```python
from build123d import *

# Parameters (mm, degrees)
AUFSATZ_LINEAR_AUSTRAGEN1_DEPTH             = 350
AUFSATZ_LINEAR_AUSTRAGEN1_DEPTH_BACK        = 350
SKIZZE1_W                                   = 200
SKIZZE1_H                                   = 2166
VERRUNDUNG1_R                               = 400
SKIZZE2_W                                   = 450
SKIZZE2_H                                   = 1500
SCHNITT_LINEAR_AUSTRAGEN1_DEPTH             = 200
SKIZZE4_W                                   = 80
SKIZZE4_H                                   = 1500
SCHNITT_LINEAR_AUSTRAGEN2_DEPTH             = 40
SKIZZE5_R                                   = 40
AUFSATZ_LINEAR_AUSTRAGEN2_DEPTH             = 1500
VERRUNDUNG2_R                               = 10
SKIZZE6_W                                   = 30
SKIZZE6_H                                   = 500
AUFSATZ_LINEAR_AUSTRAGEN3_DEPTH             = 500
SKIZZE7_W                                   = 1200
SKIZZE7_H                                   = 700
AUFSATZ_LINEAR_AUSTRAGEN4_DEPTH             = 10
SCHNITT_LINEAR_AUSTRAGEN3_DEPTH             = 2352.164614527
SCHNITT_LINEAR_AUSTRAGEN4_REACH             = 2264.149
SKIZZE10_W                                  = 160
SKIZZE10_H                                  = 700
SCHNITT_LINEAR_AUSTRAGEN4_DIRECTION_2_DEPTH = 2263.148932027


with BuildPart() as part:
    # Skizze1 → Aufsatz-Linear austragen1 (new, two sides: drawn at the far end of the back side and taken through both)
    with BuildSketch(Plane.XY.offset(-AUFSATZ_LINEAR_AUSTRAGEN1_DEPTH_BACK)):
        with Locations((0, 1083)):
            Rectangle(SKIZZE1_W, SKIZZE1_H)
    extrude(amount=AUFSATZ_LINEAR_AUSTRAGEN1_DEPTH + AUFSATZ_LINEAR_AUSTRAGEN1_DEPTH_BACK)

    # Verrundung1
    # the kernel refuses this fillet: 400 mm, written as the material it takes off along each edge
    with BuildSketch(Plane(origin=(1100, 2166, -350), x_dir=(0, -1, 0), z_dir=(-1, 0, 0)), Plane(origin=(1100, 2166, 350), x_dir=(0, 0, -1), z_dir=(-1, 0, 0))) as verrundung1_piece_1:
        with BuildLine():
            CenterArc((VERRUNDUNG1_R, VERRUNDUNG1_R), VERRUNDUNG1_R, 180, 90)
            Line((0, VERRUNDUNG1_R), (0, 0))
            Line((0, 0), (VERRUNDUNG1_R, 0))
        make_face()
    extrude(amount=2200, mode=Mode.SUBTRACT)

    # Skizze2 → Schnitt-Linear austragen1 (cut)
    with BuildSketch(Plane(origin=(100, 0, 0), x_dir=(0, 0, -1), z_dir=(1, 0, 0))):
        with Locations((0, 1050)):
            Rectangle(SKIZZE2_W, SKIZZE2_H)
    extrude(amount=-SCHNITT_LINEAR_AUSTRAGEN1_DEPTH, mode=Mode.SUBTRACT)

    # Skizze4 → Schnitt-Linear austragen2 (cut)
    with BuildSketch(Plane.XY.offset(-225)):
        with Locations((0, 1050)):
            Rectangle(SKIZZE4_W, SKIZZE4_H)
    schnitt_linear_austragen2 = extrude(amount=-SCHNITT_LINEAR_AUSTRAGEN2_DEPTH, mode=Mode.SUBTRACT)

    # Spiegeln1: Schnitt-Linear austragen2 across plane
    add(schnitt_linear_austragen2.mirror(Plane.XY), mode=Mode.SUBTRACT)

    # Skizze5 → Aufsatz-Linear austragen2 (add)
    with BuildSketch(Plane(origin=(0, 300, 0), x_dir=(1, 0, 0), z_dir=(0, 1, 0))):
        with Locations(Location((0, 0, 0), (0, 0, 90))):
            Circle(SKIZZE5_R)
    extrude(amount=AUFSATZ_LINEAR_AUSTRAGEN2_DEPTH)

    # Verrundung2
    verrundung2_edges = [part.edges().sort_by_distance(p)[0] for p in [
        (0, 300, 40),
        (0, 1800, 40),
    ]]
    fillet(verrundung2_edges, radius=VERRUNDUNG2_R)

    # Skizze6 → Aufsatz-Linear austragen3 (add)
    with BuildSketch(Plane(origin=(100, 0, 0), x_dir=(0, 0, -1), z_dir=(1, 0, 0))):
        with Locations((-335, 250)):
            Rectangle(SKIZZE6_W, SKIZZE6_H)
        with Locations((335, 250)):
            Rectangle(SKIZZE6_W, SKIZZE6_H)
    aufsatz_linear_austragen3 = extrude(amount=AUFSATZ_LINEAR_AUSTRAGEN3_DEPTH)

    # Spiegeln2: Aufsatz-Linear austragen3 across plane
    add(aufsatz_linear_austragen3.mirror(Plane(origin=(0, 0, 0), x_dir=(0, 0, 1), z_dir=(1, 0, 0))))

    # Skizze7 → Aufsatz-Linear austragen4 (add)
    with BuildSketch(Plane.XZ):
        Rectangle(SKIZZE7_W, SKIZZE7_H)
    extrude(amount=-AUFSATZ_LINEAR_AUSTRAGEN4_DEPTH)

    # Skizze9 → Schnitt-Linear austragen3 (cut, symmetric)
    with BuildSketch(Plane.XY.offset(350)):
        with BuildLine():
            Line((100, 5456.908143316), (100, 500))
            ThreePointArc((100, 500), (246.446609407, 146.446609407), (600, 0))
            Line((600, 0), (5556.908143316, 0))
            Line((5556.908143316, 0), (12567.034867032, 7010.126723715))
            Line((12567.034867032, 7010.126723715), (7110.126723715, 12467.034867032))
            Line((7110.126723715, 12467.034867032), (100, 5456.908143316))
        make_face()
    schnitt_linear_austragen3 = extrude(amount=SCHNITT_LINEAR_AUSTRAGEN3_DEPTH, both=True, mode=Mode.SUBTRACT)

    # Spiegeln3: Schnitt-Linear austragen3 across plane
    add(schnitt_linear_austragen3.mirror(Plane(origin=(0, 0, 0), x_dir=(0, 0, 1), z_dir=(1, 0, 0))), mode=Mode.SUBTRACT)

    # Schnitt-Linear austragen4: up to this face of the body (flat: up to its plane)
    schnitt_linear_austragen4_end = Plane(part.part.faces().sort_by_distance((0, 0, 0))[0])
    # Skizze10 → Schnitt-Linear austragen4 (cut, up to the picked face)
    with BuildSketch(Plane(origin=(0, 10, 0), x_dir=(1, 0, 0), z_dir=(0, 1, 0)), mode=Mode.PRIVATE) as schnitt_linear_austragen4_sk1:
        with Locations((520, 0)):
            Rectangle(SKIZZE10_W, SKIZZE10_H)
    schnitt_linear_austragen4_tool1 = split(extrude(schnitt_linear_austragen4_sk1.sketch, amount=-SCHNITT_LINEAR_AUSTRAGEN4_REACH, mode=Mode.PRIVATE), bisect_by=schnitt_linear_austragen4_end, keep=Keep.BOTH, mode=Mode.PRIVATE)
    schnitt_linear_austragen4 = schnitt_linear_austragen4_tool1.solids().sort_by(Axis((520, 10, 0), (0, -1, 0)))[0]
    add(schnitt_linear_austragen4, mode=Mode.SUBTRACT)

    # Skizze10 → Schnitt-Linear austragen4 direction 2 (cut)
    with BuildSketch(Plane(origin=(0, 10, 0), x_dir=(1, 0, 0), z_dir=(0, 1, 0))):
        with Locations((520, 0)):
            Rectangle(SKIZZE10_W, SKIZZE10_H)
    schnitt_linear_austragen4_direction_2 = extrude(amount=SCHNITT_LINEAR_AUSTRAGEN4_DIRECTION_2_DEPTH, mode=Mode.SUBTRACT)

    # Spiegeln4: Schnitt-Linear austragen4, Schnitt-Linear austragen4 direction 2 across plane
    add(schnitt_linear_austragen4.mirror(Plane(origin=(0, 0, 0), x_dir=(0, 0, 1), z_dir=(1, 0, 0))), mode=Mode.SUBTRACT)
    add(schnitt_linear_austragen4_direction_2.mirror(Plane(origin=(0, 0, 0), x_dir=(0, 0, 1), z_dir=(1, 0, 0))), mode=Mode.SUBTRACT)


solid = part.part
```
The model under review builds one solid part; all positions refer to its coordinate system, in mm. A direction names the side the tool comes from. Round coordinates to 2 decimals unless told otherwise and drop trailing zeros. Write each loop counter-clockwise with the first axis right and the second up, starting at its lowest first coordinate (ties: lowest second). Pieces come first, ordered by that corner, then holes. Notation, with made-up numbers: (86.25, -38) - (135.25, -38) arc R21 cw to (135.25, -34) - close; hole circle Ø9 at (7.25, -34). An arc over 180 degrees is marked (long way). One line per question, with ' | ' between items.
Item 1: For P1, Ø12, axis at y = 1293, z = 237, coming from the +X side; P2, Ø1.5, axis at y = 1829.5, z = 102, coming from the -X side; P3, Ø4, axis at x = -342.5, z = 16.5, coming from the +Y side, all flat-tipped, find the tip position at first contact; note any pin that passes through.
Resolved:
P1: stops at x = 100 | P2: stops at x = -100 | P3: stops at y = 10
Item 2: Add section A-A, the plane y = 944.5. Give the boundary of the cut face in (x, z), then the cut area to 3 significant figures.
Resolved:
outline: (-100, -350) - (100, -350) - (100, -225) - (40, -225) - (40, -265) - (-40, -265) - (-40, -225) - (-100, -225) - close; (-100, 225) - (-40, 225) - (-40, 265) - (40, 265) - (40, 225) - (100, 225) - (100, 350) - (-100, 350) - close; circle Ø80 at (0, 0) | area: 48,600 mm2
Item 3: Add section B-B, the plane x = 0. Give the boundary of the cut face in (y, z), then the cut area to 3 significant figures.
Resolved:
outline: (0, -350) - (1766, -350) arc R400 ccw to (2162.86, 0) arc R400 ccw to (1766, 350) - (0, 350) - close; hole (300, -265) - (1800, -265) - (1800, -50) arc R10 ccw to (1790, -40) - (310, -40) arc R10 ccw to (300, -50) - close; hole (300, 50) arc R10 ccw to (310, 40) - (1790, 40) arc R10 ccw to (1800, 50) - (1800, 265) - (300, 265) - close | area: 773,000 mm2
Item 4: Add section D-D, the plane z = 161. Give the boundary of the cut face in (x, y).
Resolved:
outline: (-440, 0) - (440, 0) - (440, 10) - (100, 10) - (100, 300) - (-100, 300) - (-100, 10) - (-440, 10) - close; (-100, 1800) - (100, 1800) - (100, 2105.82) - (-100, 2105.82) - close
Item 5: The part is to be moulded in two halves that separate along Y. For faces 1 (the face through (31, 756, -350)), 2 (the face through (191.273, 212.004, -334.79)), 3 (the face through (-1, 1060, -265)), say which applies: pulls with the +Y half, pulls with the -Y half, needs draft (parallel to the pull), parting line crosses it, or undercut.
Resolved:
face 1: needs draft | face 2: pulls with the +Y half | face 3: undercut
Item 6: To check wall thickness, follow probe 1 along Y at (x, z) = (397.5, -223); probe 2 along X at (y, z) = (1159, -317); probe 3 along Y at (x, z) = (-23, 79). State the ranges of each line that lie inside material, in increasing order.
Resolved:
probe 1: y = 0 to 10 | probe 2: x = -100 to 100 | probe 3: y = 0 to 300, 1800 to 2144.63
Item 7: For faces 4 (the face through (70, 1040, 225)), 5 (the face through (194, 127, 320)), 6 (the face through (1, 300, -55)), list the 3-axis set-ups (+Z, -Z, +X, -X, +Y, -Y) from which the entire face can be reached by the end or side of a thin tool; tool diameter is ignored.
Resolved:
face 4: +X, -X | face 5: +X, +Y | face 6: none
Item 8: Add section C-C, the plane z = -85.5. Give the boundary of the cut face in (x, y), then the cut area to 3 significant figures.
Resolved:
outline: (-440, 0) - (440, 0) - (440, 10) - (100, 10) - (100, 300) - (-100, 300) - (-100, 10) - (-440, 10) - close; (-100, 1800) - (100, 1800) - (100, 2142.35) - (-100, 2142.35) - close | area: 135,000 mm2
